The listing builds one solid part. Answer for the finished solid, in the listing's coordinates (mm). Face numbers are marked on the shaded views. A direction names the side the tool comes from. Coordinates: 2 decimals unless noted, no trailing zeros. Write each loop counter-clockwise with the first axis right and the second up, starting at its lowest first coordinate (ties: lowest second). Pieces come first, ordered by that corner, then holes. Notation, with made-up numbers: M 21.25,30.5 L 63.25,30.5 A26 cw 63.25,62.5 Z; hole C -38,-5.5 d9. An arc over 180 degrees is marked long. Write item = value, one per line. Start each with the question number.
```python
from build123d import *

# Parameters (mm, degrees)
SKETCH1_R           = 1
BOSS_EXTRUDE1_DEPTH = 6.35
SKETCH2_R           = 1
SKETCH2_W           = 13.9
SKETCH2_H           = 24
CUT_EXTRUDE1_DEPTH  = 102.470796291
FILLET1_R           = 0.5
FILLET2_R           = 2
SKETCH3_R           = 6.5
CUT_EXTRUDE2_DEPTH  = 6.35
SKETCH4_R           = 7.5
CUT_EXTRUDE3_DEPTH  = 102.470796291


with BuildPart() as part:
    # Sketch1 → Boss-Extrude1 (new body)
    with BuildSketch(Plane.XY):
        with BuildLine():
            Line((-10, 12.489995997), (-10, 100))
            Line((-10, 100), (10, 100))
            Line((10, 100), (10, 12.489995997))
            ThreePointArc((10, 12.489995997), (0, -16), (-10, 12.489995997))
        make_face()
        with Locations((-10.5, 0)):
            Circle(SKETCH1_R, mode=Mode.SUBTRACT)
        with Locations((0, 10.5)):
            Circle(SKETCH1_R, mode=Mode.SUBTRACT)
        with Locations((10.5, 0)):
            Circle(SKETCH1_R, mode=Mode.SUBTRACT)
        with Locations((0, -10.5)):
            Circle(SKETCH1_R, mode=Mode.SUBTRACT)
    extrude(amount=BOSS_EXTRUDE1_DEPTH)

    # Sketch2 → Cut-Extrude1 (cut, through all)
    with BuildSketch(Plane.XY.offset(6.35)):
        with Locations((0, 93.85)):
            Circle(SKETCH2_R)
        with Locations((0, 66.15)):
            Circle(SKETCH2_R)
        with Locations((0, 80)):
            Rectangle(SKETCH2_W, SKETCH2_H)
    extrude(amount=-CUT_EXTRUDE1_DEPTH, mode=Mode.SUBTRACT)

    # Fillet1
    fillet1_edges = [part.edges().sort_by_distance(p)[0] for p in [
        (6.95, 68, 3.175),
        (-6.95, 68, 3.175),
        (-6.95, 92, 3.175),
        (6.95, 92, 3.175),
    ]]
    fillet(fillet1_edges, radius=FILLET1_R)

    # Fillet2
    fillet2_edges = [part.edges().sort_by_distance(p)[0] for p in [
        (-10, 12.489995997, 3.175),
        (-10, 100, 3.175),
        (10, 100, 3.175),
        (10, 12.489995997, 3.175),
    ]]
    fillet(fillet2_edges, radius=FILLET2_R)

    # Sketch3 → Cut-Extrude2 (cut)
    with BuildSketch(Plane.XY.offset(6.35)):
        with Locations((0, 38.325)):
            Circle(SKETCH3_R)
        with Locations((0, 54.325)):
            Circle(SKETCH3_R)
        with Locations((0, 22.325)):
            Circle(SKETCH3_R)
    extrude(amount=-CUT_EXTRUDE2_DEPTH, mode=Mode.SUBTRACT)

    # Sketch4 → Cut-Extrude3 (cut, through all)
    with BuildSketch(Plane.XY.offset(6.35)):
        Circle(SKETCH4_R)
    extrude(amount=-CUT_EXTRUDE3_DEPTH, mode=Mode.SUBTRACT)


solid = part.part
```
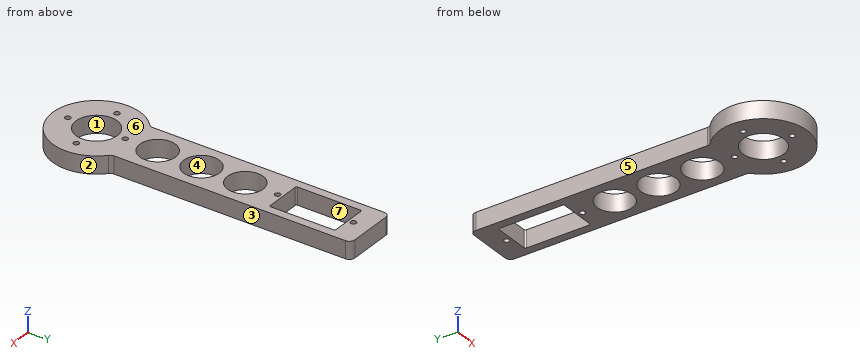
1. The part is cut by section B-B, the plane y = 0. Write down the section's boundary in (x, z).
2. For a pull along Y with two mould halves and no side action, classify the marked faces 1, 2, 3 and 4 as pulls with the +Y half, pulls with the -Y half, needs draft (parallel to the pull), parting line crosses it, or undercut.
3. For the marked faces 5, 6 and 7, determine the directions among +Z, -Z, +X, -X, +Y, -Y from which every point of the face is accessible in a straight line to the end or side of a thin tool.
4. The part is cut by section C-C, the plane z = 3. Count the separate pieces of the cut face and the enclosed holes in it, and give its area (3 significant figures).
5. The part is cut by section D-D, the plane y = 25.5. Write down the section's boundary in (x, z).
6. This flat-tipped pin is pushed along its axis until it touches: pin 1 (3 mm diameter, centred on y = 78, z = 3, fed in from -X). Where does it stop, or does it pass through?
7. Straight lines are drawn through the part: L1, parallel to Y at x = -1.5, z = 5.75; L2, parallel to Y at x = 5, z = 6.25; L3, parallel to X at y = 93.85, z = 3.25. For each, find the intervals that lie inside material, in ascending order. Write a range as [from, to].
8. The part is cut by section A-A, the plane x = 2. Write down the section's boundary in (y, z).
Solution:
q1.outline = M -16,0 L -11.5,0 L -11.5,6.35 L -16,6.35 Z; M -9.5,0 L -7.5,0 L -7.5,6.35 L -9.5,6.35 Z; M 7.5,0 L 9.5,0 L 9.5,6.35 L 7.5,6.35 Z; M 11.5,0 L 16,0 L 16,6.35 L 11.5,6.35 Z
q2.face_1 = undercut
q2.face_2 = parting line crosses it
q2.face_3 = needs draft
q2.face_4 = undercut
q3.face_5 = +Z, -Z, -X, +Y
q3.face_6 = +Z, +X, -X, +Y, -Y
q3.face_7 = +Z, -Z
q4.separate_pieces = 1
q4.enclosed_holes = 11
q4.area = 1,580 mm^2
q5.outline = M -10,0 L -5.67,0 L -5.67,6.35 L -10,6.35 Z; M 5.67,0 L 10,0 L 10,6.35 L 5.67,6.35 Z
q6.pin_1 = -10
q7.L1 = [-15.93, -7.35], [7.35, 16], [28.65, 32], [44.65, 48], [60.65, 68], [92, 100]
q7.L2 = [-15.2, -5.59], [5.59, 18.17], [26.48, 34.17], [42.48, 50.17], [58.48, 68], [92, 100]
q7.L3 = [-10, -1], [1, 10]
q8.outline = M -15.87,0 L -7.23,0 L -7.23,6.35 L -15.87,6.35 Z; M 7.23,0 L 16.14,0 L 16.14,6.35 L 7.23,6.35 Z; M 28.51,0 L 32.14,0 L 32.14,6.35 L 28.51,6.35 Z; M 44.51,0 L 48.14,0 L 48.14,6.35 L 44.51,6.35 Z; M 60.51,0 L 68,0 L 68,6.35 L 60.51,6.35 Z; M 92,0 L 100,0 L 100,6.35 L 92,6.35 Z
